For this review, take the finished solid that the model builds, in its own axes (mm). Face numbers are marked on the shaded views. A direction names the side the tool comes from. Coordinates: 2 decimals unless noted, no trailing zeros. Loops run counter-clockwise (first coordinate to the right, second up) from the corner with the lowest first, then second, coordinate; pieces in that order, holes last. Notation, with made-up numbers: M 4.5,37 L 63.5,37 A14 ccw 63.5,61 Z; hole C 6.25,-35 d3. An arc over 180 degrees is marked long. Write item = value, one per line.
Autodesk Inventor part; units mm, degrees
ref_plane "YZ Plane" through (0, 0, 0) normal (1, 0, 0) x (0, 1, 0)
ref_plane "XZ Plane" through (0, 0, 0) normal (0, 1, 0) x (-1, 0, 0)
ref_plane "XY Plane" through (0, 0, 0) normal (0, 0, 1) x (1, 0, 0)
sketch "Sketch1" plane through (0, 0, 0) normal (0, 0, 1) x (1, 0, 0)
  circle A0 centre (4, 4) radius 1.2
  circle A1 centre (4, 4) radius 1.5
  point P0 (0, 0)
  dimension "d0" = 3
extrude "Extrusion1" add sketch "Sketch1" against normal blind 15 contours A0 | A1
sketch "Sketch2" plane through (4, 4, 0) normal (0, 0, 1) x (1, 0, 0)
  circle A0 centre (0, 0) radius 1.5
  circle A1 centre (0, 0) radius 2.8
  point P0 (-4, -4)
  dimension "d3" = 5.6
extrude "Extrusion2" add sketch "Sketch2" along normal blind 3 contours A0 | A1
fillet "Fillet1" radius 0.3 1 edges at (1.2, 4, 3)
sketch "Sketch3" plane through (4, 4, 0) normal (0, 0, -1) x (-1, 0, 0)
  circle A0 centre (0, 0) radius 2.8
  circle A1 centre (0, 0) radius 1.5
  circle A2 centre (0, 0) radius 2.75
  point P0 (4, -4)
  dimension "d7" = 5.5
extrude "Extrusion3" cut sketch "Sketch3" against normal blind 0.5 contours A0
sketch "Sketch4" plane through (4, 4, 3) normal (0, 0, 1) x (1, 0, 0)
  circle A0 centre (0, 0) radius 2.5
  line L0 (0.7217, 1.25) -> (1.4434, 0)
  line L1 (1.4434, 0) -> (0.7217, -1.25)
  line L2 (0.7217, -1.25) -> (-0.7217, -1.25)
  line L3 (-0.7217, -1.25) -> (-1.4434, 0)
  line L4 (-1.4434, 0) -> (-0.7217, 1.25)
  line L5 (-0.7217, 1.25) -> (0.7217, 1.25)
  point P0 (-4, -4)
  dimension "d10" = 2.5
extrude "Extrusion4" cut sketch "Sketch4" against normal blind 2 contours L0 L1 L2 L3 L4 L5
thread "Thread1"
properties part number "m3 6" material "Steel"
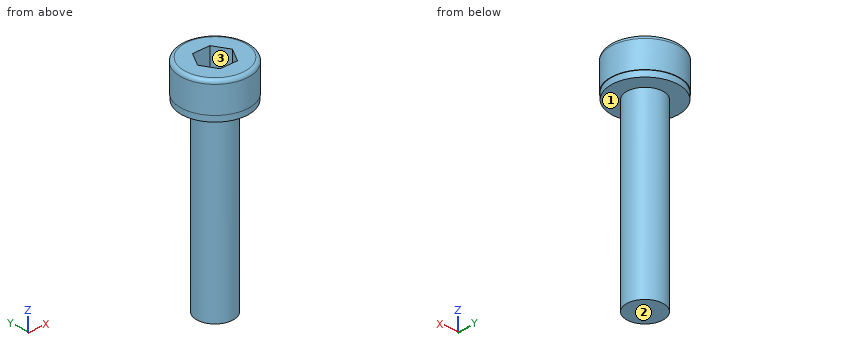
Q1. For line 1 along Z through (x, y) = (2.1, 4.2); line 2 along X through (y, z) = (4.4, -5.5); line 3 along Y through (x, z) = (3.95, -7.5), list the stretches that pass through material, from the lowest coordinate up.
Solved:
line_1 = 0 to 3
line_2 = 2.55 to 5.45
line_3 = 2.5 to 5.5
Q2. Add section A-A (x = 4). Write out the cut boundary in (y, z), and give its area (3 significant figures).
Solved:
outline = M 1.2,0.5 L 1.25,0.5 L 1.25,0 L 2.5,0 L 2.5,-15 L 5.5,-15 L 5.5,0 L 6.75,0 L 6.75,0.5 L 6.8,0.5 L 6.8,2.7 A0.3 ccw 6.5,3 L 5.25,3 L 5.25,1 L 2.75,1 L 2.75,3 L 1.5,3 A0.3 ccw 1.2,2.7 Z
area = 56.7 mm²
Q3. For pin 1 Ø0.8 at (x, y) = (4.5, 4.5) entering from +Z; pin 2 Ø1.2 at (x, z) = (3.5, 2) entering from -Y; pin 3 Ø1.5 at (y, z) = (3.5, -13) entering from -X, all flat-tipped, find the tip position at first contact; note any pin that passes through.
Solved:
pin_1 = 1
pin_2 = 1.2
pin_3 = 2.5
Q4. Add section B-B (z = -11). Write out the cut boundary in (x, y).
Solved:
outline = C 4,4 d3
Q5. Machinability: for the marked faces 1, 2 and 3, which of the approach directions +Z, -Z, +X, -X, +Y, -Y give a long, thin tool a straight path to every point of the face, cutting with its end or side? Answer none if there is none.
Solved:
face_1 = -Z
face_2 = -Z, +X, -X, +Y, -Y
face_3 = +Z
